Source: CAD feature listing. Evaluate the final solid. Frame: model axes, mm. A direction names the side the tool comes from. Give positions to 0.01 mm unless a question says otherwise; leave off trailing zeros. Order: outer loops, then holes, each group sorted by start corner. A loop starts at its lowest first (then second) coordinate and runs counter-clockwise, first axis right, second up. Notation, with made-up numbers: M -26.75,68 L 32.25,68 A12 cw 32.25,91 Z; hole C 84.25,14.25 d4. An arc over 180 degrees is marked long. Answer as a JSON object with one key per item and string values. Group by question number.
1. Pin query (flat end, axial travel): P1, Ø2.5, axis at y = 1, z = 19.5, coming from the +X side; P2, Ø6.5, axis at y = 4, z = -5.5, coming from the +X side; P3, Ø4, axis at y = 38, z = -1, coming from the +X side. Return the tip coordinate at first contact, or that it passes through.
2. Section query C-C (y = 9). Output: boundary loops of the cut face in (x, z), plus the area to 3 significant figures.
3. Section query D-D (x = 15.5). Output: boundary loops of the cut face in (y, z).
4. Material intervals for L1, parallel to Z at x = 15.5, y = 4.7; L2, parallel to Z at x = -15.5, y = 1.6; L3, parallel to Z at x = 13, y = 15.5, sorted ascending. Write a range as [from, to].
5. Section query A-A (x = -15.5). Output: boundary loops of the cut face in (y, z), plus the area to 3 significant figures.
6. Set-up query: faces 1 (the flat face through (-16, 6, 0)), 2 (the flat face through (-12.35, 3, 0)), 3 (the cylindrical face through (17.07, 3.04, -14.85)). Return all of +Z, -Z, +X, -X, +Y, -Y with unobstructed straight access to the full face (end or side cutting, diameter ignored); none if empty.
7. Section query B-B (z = -18.5). Output: boundary loops of the cut face in (x, y).
8. Pull-direction query (Z, two-part tool) for faces 4 (the flat face through (0, 29, 28.5)), 5 (the cylindrical face through (27.07, 61.5, -0.33)), 6 (the flat face through (-22.5, 32, 0)); classes: +Z half, -Z half, draft (parallel to the pull), parting line (faces both ways), or undercut.
from build123d import *

# Parameters (mm, degrees)
SKETCH1_W                 = 57
SKETCH1_H                 = 57
BOSS_EXTRUDE3_DEPTH       = 63
SKETCH3_W                 = 45
SKETCH3_H                 = 57
CUT_EXTRUDE2_DEPTH        = 29.5
CUT_EXTRUDE2_DEPTH_BACK   = 22.5
BOSS_EXTRUDE4_DEPTH       = 6
F_5_0MM_DOWEL_HOLE1_D     = 3.4
F_5_0MM_DOWEL_HOLE1_DEPTH = 6
F_5_0MM_DOWEL_HOLE1_TIP   = 1.021463052
FILLET1_R                 = 5
FILLET2_R                 = 3


with BuildPart() as part:
    # Sketch1 → Boss-Extrude3 (new body)
    with BuildSketch(Plane(origin=(0, 0, 0), x_dir=(1, 0, 0), z_dir=(0, 1, 0))):
        Rectangle(SKETCH1_W, SKETCH1_H)
    extrude(amount=BOSS_EXTRUDE3_DEPTH)

    # Sketch3 → Cut-Extrude2 (cut, two sides)
    with BuildSketch(Plane(origin=(0, 0, 0), x_dir=(0, 0, -1), z_dir=(1, 0, 0))) as cut_extrude2_sk:
        with Locations((0, 28.5)):
            Rectangle(SKETCH3_W, SKETCH3_H)
    extrude(amount=CUT_EXTRUDE2_DEPTH, mode=Mode.SUBTRACT)
    extrude(cut_extrude2_sk.sketch, amount=-CUT_EXTRUDE2_DEPTH_BACK, mode=Mode.SUBTRACT)

    # Sketch1<6> → Boss-Extrude4 (add)
    with BuildSketch(Plane(origin=(0, 0, 0), x_dir=(1, 0, 0), z_dir=(0, 1, 0))):
        Polygon((22.5, 22.5), (-22.5, 22.5), (-22.5, -22.5), (22.5, -22.5), (22.5, -12.350491759), (-12.350491759, -12.350491759), (-12.350491759, 12.350491759), (22.5, 12.350491759), align=None)
    extrude(amount=BOSS_EXTRUDE4_DEPTH)

    # Ø5.0mm Dowel Hole1
    with Locations(Plane(origin=(0, 0, 0), x_dir=(-1, 0, 0), z_dir=(0, -1, 0))):
        with Locations((15.5, -15.5), (15.5, 15.5), (-15.5, 15.5), (-15.5, -15.5)):
            Hole(F_5_0MM_DOWEL_HOLE1_D / 2, depth=F_5_0MM_DOWEL_HOLE1_DEPTH)
            with Locations((0, 0, -(F_5_0MM_DOWEL_HOLE1_DEPTH + F_5_0MM_DOWEL_HOLE1_TIP / 2))):  # 118° drill point
                Cone(0, F_5_0MM_DOWEL_HOLE1_D / 2, F_5_0MM_DOWEL_HOLE1_TIP, mode=Mode.SUBTRACT)

    # Fillet1
    fillet1_edges = [part.edges().sort_by_distance(p)[0] for p in [
        (0, 63, -28.5),
        (-28.5, 63, 0),
        (0, 63, 28.5),
        (28.5, 63, 0),
        (28.5, 31.5, 28.5),
        (-28.5, 31.5, 28.5),
        (-28.5, 31.5, -28.5),
        (28.5, 31.5, -28.5),
    ]]
    fillet(fillet1_edges, radius=FILLET1_R)

    # Fillet2
    fillet2_edges = [part.edges().sort_by_distance(p)[0] for p in [
        (22.5, 6, -17.425245879),
        (22.5, 6, 17.425245879),
    ]]
    fillet(fillet2_edges, radius=FILLET2_R)


solid = part.part
Answer sheet:
{
 "1": {"P1": "x = 22.5", "P2": "x = -12.35", "P3": "x = -22.5"},
 "2": {"outline": "M -28.5,-23.5 A5 ccw -23.5,-28.5 L 23.5,-28.5 A5 ccw 28.5,-23.5 L 28.5,-22.5 L -22.5,-22.5 L -22.5,22.5 L 28.5,22.5 L 28.5,23.5 A5 ccw 23.5,28.5 L -23.5,28.5 A5 ccw -28.5,23.5 Z", "area": "933 mm^2"},
 "3": {"outline": "M 0,-28.5 L 58,-28.5 A5 ccw 63,-23.5 L 63,23.5 A5 ccw 58,28.5 L 0,28.5 L 0,17.2 L 6,17.2 L 6,22.5 L 57,22.5 L 57,-22.5 L 6,-22.5 L 6,-17.2 L 0,-17.2 Z; M 0,-13.8 L 6,-13.8 L 6,-12.35 L 0,-12.35 Z; M 0,12.35 L 6,12.35 L 6,13.8 L 0,13.8 Z"},
 "4": {"L1": "[-28.5, -17.2], [-13.8, -12.35], [12.35, 13.8], [17.2, 28.5]", "L2": "[-28.5, -17.2], [-13.8, 13.8], [17.2, 28.5]", "L3": "[-28.5, -22.5], [22.5, 28.5]"},
 "5": {"outline": "M 0,-28.5 L 58,-28.5 A5 ccw 63,-23.5 L 63,23.5 A5 ccw 58,28.5 L 0,28.5 L 0,17.2 L 6,17.2 L 6,22.5 L 57,22.5 L 57,-22.5 L 6,-22.5 L 6,-17.2 L 0,-17.2 Z; M 0,-13.8 L 6,-13.8 L 6,13.8 L 0,13.8 Z", "area": "1,240 mm^2"},
 "6": {"face 1": "+X", "face 2": "+X, -Y", "face 3": "-Y"},
 "7": {"outline": "M -28.5,0 L 22.5,0 L 22.5,3 A3 ccw 19.5,6 L -22.5,6 L -22.5,57 L 28.5,57 L 28.5,58 A5 ccw 23.5,63 L -23.5,63 A5 ccw -28.5,58 Z"},
 "8": {"face 4": "+Z half", "face 5": "draft", "face 6": "undercut"}
}
